Source: CAD feature listing. Evaluate the final solid. Frame: model axes, mm. Face numbers are marked on the shaded views. A direction names the side the tool comes from. Give positions to 0.01 mm unless a question says otherwise; leave off trailing zeros. Write each loop counter-clockwise with the first axis right and the second up, starting at its lowest first coordinate (ties: lowest second). Pieces come first, ordered by that corner, then holes. Notation, with made-up numbers: (48, -23) -> (62, -23) arc R26 ccw to (62, -3) -> close; hole circle Ø3 at (-25.75, 12). An arc over 180 degrees is marked (long way). Use one line per item in the form item = value. Start each with the question number.
(1) Cut plane A-A, the plane z = 0. Output: boundary loops of the cut face in (x, y), and give its area (3 significant figures).
(2) Cut plane B-B, the plane x = -18. Output: boundary loops of the cut face in (y, z).
(3) Set-up query: the marked faces 1 and 2. Return all of +Z, -Z, +X, -X, +Y, -Y with unobstructed straight access to the full face (end or side cutting, diameter ignored); none if empty.
(4) Cut plane D-D, the plane x = 0. Output: boundary loops of the cut face in (y, z).
(5) Material intervals for line 1 along X through (y, z) = (11.75, 5.25); line 2 along Z through (x, y) = (18, 8.5); line 3 along Z through (x, y) = (-18, 1.3), sorted ascending. Write a range as from..to.
(6) First-contact query: P1, Ø4, axis at x = -17, z = 0, coming from the -Y side; P2, Ø2, axis at x = -18, z = 0, coming from the -Y side; P3, Ø4, axis at x = 2.5, y = 7.5, coming from the +Z side. Flat tips, straight axial feed; report the tip coordinate or a pass-through.
(7) Cut plane C-C, the plane y = 11. Output: boundary loops of the cut face in (x, z).
(8) Draft query along X for the marked faces 3, 4 and 5. Return one class per face: pulls with the +X half, pulls with the -X half, needs draft (parallel to the pull), parting line crosses it, or undercut.
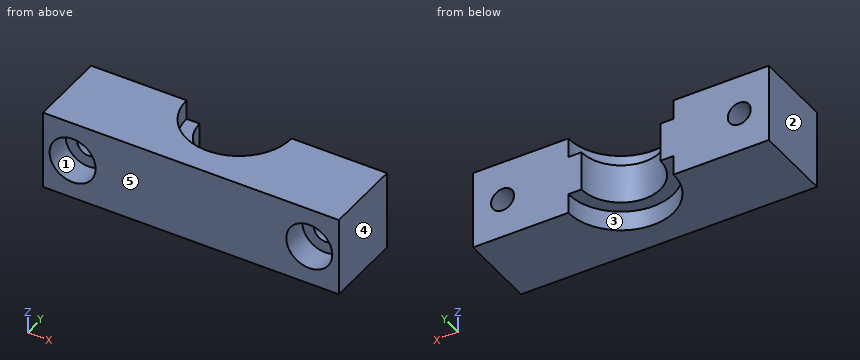
from build123d import *

# Parameters (mm, degrees)
F0_W     = 45
F0_H     = 12
F0_R     = 3.5
F0_R_2   = 1.75
F1_DEPTH = 12
F2_DEPTH = 4
F4_DEPTH = 12.001
F3_R     = 8
F3_R_2   = 6
F5_DEPTH = 3
F6_R     = 8
F7_DEPTH = 3


with BuildPart() as f1:
    # F0 (on Front) → F1 (new body)
    with BuildSketch(Plane.XZ):
        Rectangle(F0_W, F0_H)
        with Locations((-18, 0)):
            Circle(F0_R, mode=Mode.SUBTRACT)
        with Locations((18, 0)):
            Circle(F0_R, mode=Mode.SUBTRACT)
        with Locations((-18, 0)):
            Circle(F0_R)
        with Locations((-18, 0)):
            Circle(F0_R_2, mode=Mode.SUBTRACT)
        with Locations((18, 0)):
            Circle(F0_R)
        with Locations((18, 0)):
            Circle(F0_R_2, mode=Mode.SUBTRACT)
    extrude(amount=-F1_DEPTH)

    # F0 (on Front) → F2 (cut)
    with BuildSketch(Plane.XZ):
        with Locations((-18, 0)):
            Circle(F0_R)
        with Locations((-18, 0)):
            Circle(F0_R_2, mode=Mode.SUBTRACT)
        with Locations((18, 0)):
            Circle(F0_R)
        with Locations((18, 0)):
            Circle(F0_R_2, mode=Mode.SUBTRACT)
    extrude(amount=-F2_DEPTH, mode=Mode.SUBTRACT)

    # F3 (on face) → F4 (cut, through all)
    with BuildSketch(Plane.XY.offset(6)):
        with BuildLine():
            Line((-6, 12), (6, 12))
            ThreePointArc((6, 12), (0, 18), (-6, 12))
        make_face()
        with BuildLine():
            ThreePointArc((-6, 12), (0, 6), (6, 12))
            Line((6, 12), (-6, 12))
        make_face()
    extrude(amount=-F4_DEPTH, mode=Mode.SUBTRACT)

    # F3 (on face) → F5 (cut)
    with BuildSketch(Plane.XY.offset(6)):
        with Locations((0, 12)):
            Circle(F3_R)
        with Locations((0, 12)):
            Circle(F3_R_2, mode=Mode.SUBTRACT)
    extrude(amount=-F5_DEPTH, mode=Mode.SUBTRACT)

    # F6 (on face) → F7 (cut)
    with BuildSketch(Plane(origin=(0, 0, -6), x_dir=(1, 0, 0), z_dir=(0, 0, -1))):
        with Locations((0, -12)):
            Circle(F6_R)
    extrude(amount=-F7_DEPTH, mode=Mode.SUBTRACT)


solid = f1.part
Geometry says:
q1.outline = (-22.5, 0) -> (-21.5, 0) -> (-21.5, 4) -> (-19.75, 4) -> (-19.75, 12) -> (-22.5, 12) -> close; (-16.25, 4) -> (-14.5, 4) -> (-14.5, 0) -> (14.5, 0) -> (14.5, 4) -> (16.25, 4) -> (16.25, 12) -> (6, 12) arc R6 cw to (-6, 12) -> (-16.25, 12) -> close; (19.75, 4) -> (21.5, 4) -> (21.5, 0) -> (22.5, 0) -> (22.5, 12) -> (19.75, 12) -> close
q1.area = 371 mm^2
q2.outline = (0, -6) -> (12, -6) -> (12, -1.75) -> (4, -1.75) -> (4, -3.5) -> (0, -3.5) -> close; (0, 3.5) -> (4, 3.5) -> (4, 1.75) -> (12, 1.75) -> (12, 6) -> (0, 6) -> close
q3.face_1 = -Y
q3.face_2 = +Z, -Z, -X, +Y, -Y
q4.outline = (0, -6) -> (4, -6) -> (4, -3) -> (6, -3) -> (6, 3) -> (4, 3) -> (4, 6) -> (0, 6) -> close
q5.line_1 = -22.5..-8, 8..22.5
q5.line_2 = -6..-1.75, 1.75..6
q5.line_3 = -6..-3.5, 3.5..6
q6.P1 = 4
q6.P2 = through
q6.P3 = 3
q7.outline = (-22.5, -6) -> (-7.94, -6) -> (-7.94, -3) -> (-5.92, -3) -> (-5.92, 3) -> (-7.94, 3) -> (-7.94, 6) -> (-22.5, 6) -> close; (5.92, -3) -> (7.94, -3) -> (7.94, -6) -> (22.5, -6) -> (22.5, 6) -> (7.94, 6) -> (7.94, 3) -> (5.92, 3) -> close; hole circle Ø3.5 at (-18, 0); hole circle Ø3.5 at (18, 0)
q8.face_3 = undercut
q8.face_4 = pulls with the +X half
q8.face_5 = needs draft
